Model file for the job. Use its own axes, mm. A direction names the side the tool comes from. Coordinates: 2 decimals unless noted, no trailing zeros. Write each loop counter-clockwise with the first axis right and the second up, starting at its lowest first coordinate (ties: lowest second). Pieces come first, ordered by that corner, then holes.
Q1. Drill centre lines: probe 1 along X at (y, z) = (2.2, -60); probe 2 along Z at (x, y) = (2.5, 2); probe 3 along X at (y, z) = (2.75, -45). Where is each one in solid material? Low to high.
Q2. Band-saw the part on D-D, the plane z = -61.5. Write the cut outline in (x, y), plus the area to 3 significant figures.
Q3. Band-saw the part on A-A, the plane y = 3.75. Write the cut outline in (x, z).
Q4. Band-saw the part on B-B, the plane z = 2.5. Write the cut outline in (x, y).
Q5. Band-saw the part on C-C, the plane x = 6. Write the cut outline in (y, z), plus the area to 3 significant figures.
Q6. Which spindle directions (+Z, -Z, +X, -X, +Y, -Y) get a long thin tool onto all of the face, cutting with end or side? Do faces 4 (the flat face through (-25, 2, -50)), 5 (the flat face through (-6, 0, -39)). Say none if no direction does.
Q7. Pull direction X, two halves, no side cores. Call faces 1 (the flat face through (-20, 2, -70)), 2 (the cylindrical face through (0, 2, 10)), 3 (the cylindrical face through (-1.532, 2.465, -63.695)): released by +X, released by -X, zero draft, split by the parting line, or undercut.
Q8. Pin check, flat tips, straight feed: P1, Ø5, axis at x = -31, z = -48, coming from the +Y side; P2, Ø2, axis at y = 2.5, z = -25.5, coming from the -X side; P3, Ø7, axis at x = -40, z = -60, coming from the +Y side. Stop position of each tip, or through.
from build123d import *

# Parameters (mm, degrees)
BOSS_EXTRUDE1_DEPTH = 5
SKETCH2_R           = 4
CUT_EXTRUDE1_DEPTH  = 5


with BuildPart() as part:
    # Sketch1 → Boss-Extrude1 (new body)
    with BuildSketch(Plane(origin=(0, 0, 0), x_dir=(1, 0, 0), z_dir=(0, 1, 0))):
        with BuildLine():
            Line((-40, 70), (0, 70))
            ThreePointArc((0, 70), (7.071067812, 67.071067812), (10, 60))
            Line((10, 60), (10, 0))
            ThreePointArc((10, 0), (0, -10), (-10, 0))
            Line((-10, 0), (-10, 50))
            Line((-10, 50), (-40, 50))
            ThreePointArc((-40, 50), (-50, 60), (-40, 70))
        make_face()
    extrude(amount=BOSS_EXTRUDE1_DEPTH)

    # Sketch2 → Cut-Extrude1 (cut)
    with BuildSketch(Plane.XZ):
        with Locations(Location((0, 0, 0), (0, 0, 270))):
            Circle(SKETCH2_R)
        with Locations(Location((-40, -60, 0), (0, 0, 270))):
            Circle(SKETCH2_R)
        with Locations(Location((0, -60, 0), (0, 0, 270))):
            Circle(SKETCH2_R)
    extrude(amount=-CUT_EXTRUDE1_DEPTH, mode=Mode.SUBTRACT)


solid = part.part
Answer sheet:
1. probe 1: x = -50 to -44, -36 to -4, 4 to 10
1. probe 2: z = -69.68 to -63.12, -56.88 to -3.12, 3.12 to 9.68
1. probe 3: x = -10 to 10
2. outline: (-49.89, 0) - (-43.71, 0) - (-43.71, 5) - (-49.89, 5) - close; (-36.29, 0) - (-3.71, 0) - (-3.71, 5) - (-36.29, 5) - close; (3.71, 0) - (9.89, 0) - (9.89, 5) - (3.71, 5) - close
2. area: 225 mm2
3. outline: (-40, -70) - (0, -70) arc R10 ccw to (10, -60) - (10, 0) arc R10 ccw to (-10, 0) - (-10, -50) - (-40, -50) arc R10 ccw to start; hole circle Ø8 at (-40, -60); hole circle Ø8 at (0, -60); hole circle Ø8 at (0, 0)
4. outline: (-9.68, 0) - (-3.12, 0) - (-3.12, 5) - (-9.68, 5) - close; (3.12, 0) - (9.68, 0) - (9.68, 5) - (3.12, 5) - close
5. outline: (0, -68) - (5, -68) - (5, 8) - (0, 8) - close
5. area: 380 mm2
6. face 4: +Z, -X, +Y, -Y
6. face 5: +Z, -Z, +X, -X, -Y
7. face 1: zero draft
7. face 2: split by the parting line
7. face 3: undercut
8. P1: stops at y = 5
8. P2: stops at x = -10
8. P3: passes through
